Check sheet for the drawn part. Datum: minimum x, y, z corner. Units: mm. A direction names the side the tool comes from. Round coordinates to 2 decimals unless told otherwise and drop trailing zeros. Order: outer loops, then holes, each group sorted by start corner. A loop starts at its lowest first (then second) coordinate and runs counter-clockwise, first axis right, second up. Notation, with made-up numbers: (17.5, 79) - (38.5, 79) arc R16 ccw to (38.5, 105) - close; hole circle Ø5 at (41, 16). An arc over 180 degrees is marked (long way). Write each question's results on one line, items separated by ' | '.
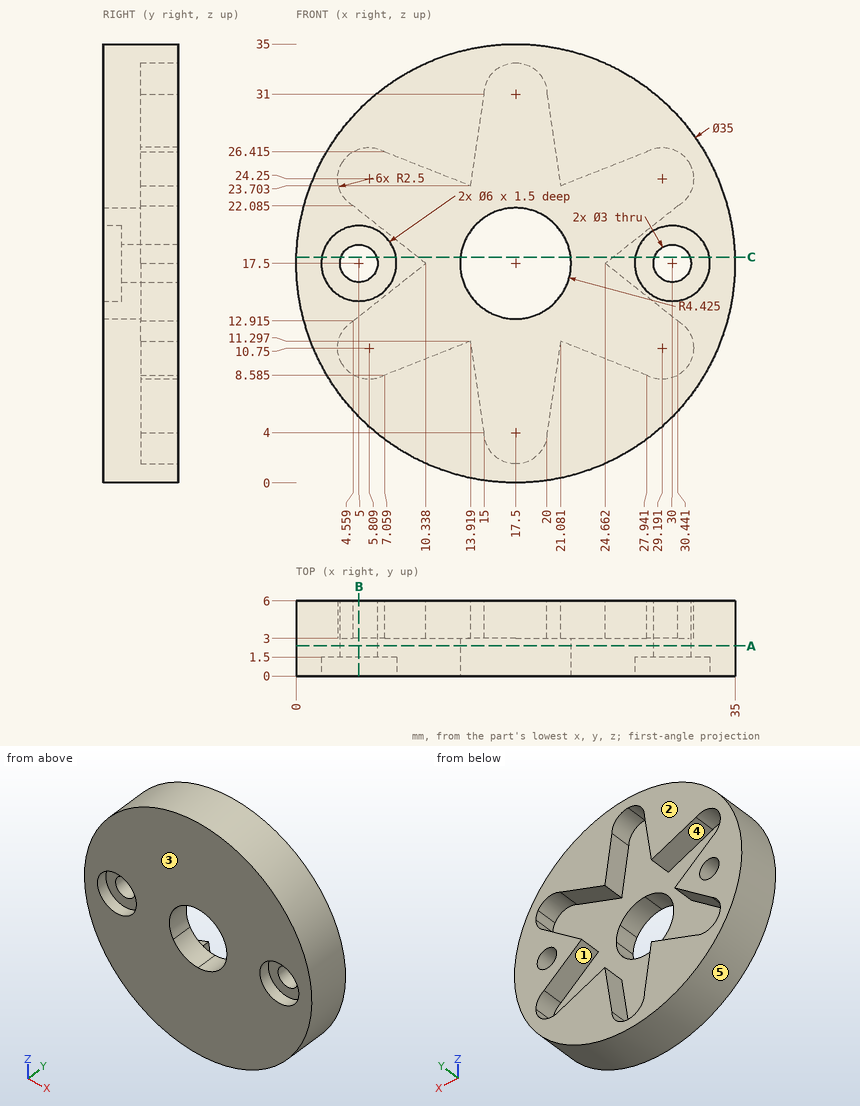
(1) Section check A-A (y = 2.4). Give the number of separate pieces and of enclosed holes in the cut face.
Answers follow:
separate pieces: 1 | enclosed holes: 3
(2) Access from +Z, -Z, +X, -X, +Y, -Y to the whole of each face (thin tool, end or side, straight path). Record for the marked faces 1 and 2.
Answers follow:
face 1: +Y | face 2: +Z, -Z, +X, -X, +Y
(3) Depth check by flat-ended pin: pin 1 Ø1.5 at (x, z) = (16, 9) entering from -Y; pin 2 Ø1.8 at (x, z) = (29, 17.5) entering from -Y; pin 3 Ø3 at (y, z) = (1.5, 28.5) entering from -X; pin 4 Ø8.5 at (x, z) = (16.5, 18) entering from +Y. Enter the tip coordinate at first touch or a pass-through.
Answers follow:
pin 1: y = 0 | pin 2: y = 1.5 | pin 3: x = 2.8 | pin 4: y = 3
(4) Draft check along Z on the marked faces 3, 4 and 5. Enter one of: released by +Z, released by -Z, zero draft, split by the parting line, or undercut.
Answers follow:
face 3: zero draft | face 4: undercut | face 5: split by the parting line
(5) Section check C-C (z = 18). Record the cut outline in (x, y).
Answers follow:
outline: (0.01, 0) - (2.04, 0) - (2.04, 1.5) - (3.59, 1.5) - (3.59, 6) - (0.01, 6) - close; (6.41, 1.5) - (7.96, 1.5) - (7.96, 0) - (13.1, 0) - (13.1, 3) - (9.71, 3) - (9.71, 6) - (6.41, 6) - close; (21.9, 0) - (27.04, 0) - (27.04, 1.5) - (28.59, 1.5) - (28.59, 6) - (25.29, 6) - (25.29, 3) - (21.9, 3) - close; (31.41, 1.5) - (32.96, 1.5) - (32.96, 0) - (34.99, 0) - (34.99, 6) - (31.41, 6) - close
(6) Material ranges on line 1 (X direction, y = 0.95, z = 17.5) (1 decimal); line 2 (X direction, y = 2.65, z = 17.5) (1 decimal); line 3 (Z direction, x = 29.5, y = 5.45) (1 decimal), recorded low to high.
Answers follow:
line 1: 0 to 2, 8 to 13.1, 21.9 to 27, 33 to 35 | line 2: 0 to 3.5, 6.5 to 13.1, 21.9 to 28.5, 31.5 to 35 | line 3: 4.8 to 8.3, 13.7 to 16.1, 18.9 to 21.3, 26.7 to 30.2
(7) Section check B-B (x = 5). Record the cut outline in (y, z) (1 decimal).
Answers follow:
outline: (0, 5.3) - (6, 5.3) - (6, 8.4) - (3, 8.4) - (3, 13.3) - (6, 13.3) - (6, 16) - (1.5, 16) - (1.5, 14.5) - (0, 14.5) - close; (0, 20.5) - (1.5, 20.5) - (1.5, 19) - (6, 19) - (6, 21.7) - (3, 21.7) - (3, 26.6) - (6, 26.6) - (6, 29.7) - (0, 29.7) - close
